Source: CAD feature listing. Evaluate the final solid. Frame: model axes, mm. Round coordinates to 2 decimals unless told otherwise and drop trailing zeros. Order: outer loops, then holes, each group sorted by start corner. A loop starts at its lowest first (then second) coordinate and runs counter-clockwise, first axis right, second up. Notation, with made-up numbers: (-28.75, -31.75) - (22.25, -31.75) arc R14 ccw to (22.25, -10.75) - close; hole circle Ø3 at (-38.75, 68.5). An arc over 180 degrees is marked (long way). Use one line per item in the form item = value. Start each with the question number.
Q1. Cut plane A-A, the plane y = 4.25. Return the cut outline in (x, z).
Q2. Ray query, line 1 (X direction, y = 16, z = -608); line 2 (Z direction, x = 79.5, y = 10.5); line 3 (X direction, y = 16.75, z = -755). Return the intervals inside material, ascending. Write a range as [from, to].
Q3. Pin query (flat end, axial travel): pin 1 Ø8 at (y, z) = (16, -914.5) entering from -X; pin 2 Ø4 at (x, z) = (-200.03, -287.05) entering from -Y; pin 3 Ø2 at (y, z) = (5.5, -580) entering from -X; pin 4 Ø8 at (x, y) = (-276.5, 5.5) entering from +Z. Return the tip coordinate at first contact, or that it passes through.
Q4. Cut plane B-B, the plane x = -234.5. Return the cut outline in (y, z).
from build123d import *

# Parameters (mm, degrees)
BOSS_EXTRUDE3_DEPTH = 19.05
SKETCH6_R           = 3.175
CUT_EXTRUDE3_DEPTH  = 9.525
CUT_EXTRUDE4_DEPTH  = 9.525


with BuildPart() as part:
    # Sketch2 → Boss-Extrude3 (new body)
    with BuildSketch(Plane(origin=(0, 0, 0), x_dir=(1, 0, 0), z_dir=(0, 1, 0))):
        Polygon((-336.69350738, 0), (-316.143895572, 0), (-209.015455166, 264.828592555), (-221.216787177, 285.466092555), align=None)
        Polygon((-316.143895572, 0), (-295.594283764, 0), (-196.814123155, 244.191092555), (-209.015455166, 264.828592555), align=None)
        with BuildLine():
            Line((-322.659375, -16.106696225), (-316.143895572, 0))
            Line((-316.143895572, 0), (-336.69350738, 0))
            Line((-336.69350738, 0), (-341.509822647, -11.90625))
            Line((-341.509822647, -11.90625), (-326.793303775, -17.859375))
            ThreePointArc((-326.793303775, -17.859375), (-325.089331047, -16.126870931), (-322.659375, -16.106696225))
        make_face()
        with BuildLine():
            Line((-303.300388192, -19.05), (-295.594283764, 0))
            Line((-295.594283764, 0), (-316.143895572, 0))
            Line((-316.143895572, 0), (-322.659375, -16.106696225))
            ThreePointArc((-322.659375, -16.106696225), (-321.217429073, -17.275121043), (-320.675, -19.05))
            Line((-320.675, -19.05), (-303.300388192, -19.05))
        make_face()
        with BuildLine():
            Line((-327.557139607, -38.1), (-311.00649262, -38.1))
            Line((-311.00649262, -38.1), (-306.190177353, -26.19375))
            Line((-306.190177353, -26.19375), (-320.906696225, -20.240625))
            ThreePointArc((-320.906696225, -20.240625), (-325.040625, -21.993303775), (-326.793303775, -17.859375))
            Line((-326.793303775, -17.859375), (-341.509822647, -11.90625))
            Line((-341.509822647, -11.90625), (-348.653572647, -29.566072647))
            Line((-348.653572647, -29.566072647), (-327.557139607, -38.1))
        make_face()
        with BuildLine():
            Line((-320.906696225, -20.240625), (-306.190177353, -26.19375))
            Line((-306.190177353, -26.19375), (-303.300388192, -19.05))
            Line((-303.300388192, -19.05), (-320.675, -19.05))
            ThreePointArc((-320.675, -19.05), (-320.733462299, -19.656479808), (-320.906696225, -20.240625))
        make_face()
        Polygon((-313.333927353, -43.853572647), (-311.00649262, -38.1), (-327.557139607, -38.1), align=None)
        Polygon((-183.626593256, 296.748681841), (-178.833212823, 288.641092555), (143.866072647, 1086.375076786), (108.546427353, 1100.662576786), (-215.267964049, 300.171976915), (-193.321682542, 313.147088585), align=None)
        with BuildLine():
            Line((-196.814123155, 244.191092555), (-187.823667989, 266.416092555))
            Line((-187.823667989, 266.416092555), (-198.409151786, 284.320524764))
            ThreePointArc((-198.409151786, 284.320524764), (-199.787821823, 283.887463765), (-201.215625, 284.11028878))
            Line((-201.215625, 284.11028878), (-209.015455166, 264.828592555))
            Line((-209.015455166, 264.828592555), (-196.814123155, 244.191092555))
        make_face()
        with BuildLine():
            Line((-197.291932209, 288.669440769), (-183.626593256, 296.748681841))
            Line((-183.626593256, 296.748681841), (-193.321682542, 313.147088585))
            Line((-193.321682542, 313.147088585), (-215.267964049, 300.171976915))
            Line((-215.267964049, 300.171976915), (-221.216787177, 285.466092555))
            Line((-221.216787177, 285.466092555), (-209.015455166, 264.828592555))
            Line((-209.015455166, 264.828592555), (-201.215625, 284.11028878))
            ThreePointArc((-201.215625, 284.11028878), (-202.431501435, 289.124673395), (-197.291932209, 288.669440769))
        make_face()
        with BuildLine():
            Line((-187.823667989, 266.416092555), (-178.833212823, 288.641092555))
            Line((-178.833212823, 288.641092555), (-183.626593256, 296.748681841))
            Line((-183.626593256, 296.748681841), (-197.291932209, 288.669440769))
            ThreePointArc((-197.291932209, 288.669440769), (-196.962475287, 287.891188748), (-196.85, 287.053592555))
            ThreePointArc((-196.85, 287.053592555), (-197.26719806, 285.480330511), (-198.409151786, 284.320524764))
            Line((-198.409151786, 284.320524764), (-187.823667989, 266.416092555))
        make_face()
    extrude(amount=BOSS_EXTRUDE3_DEPTH)

    # Sketch6 → Cut-Extrude3 (cut)
    with BuildSketch(Plane.XZ):
        Polygon((-327.557139607, 38.1), (-348.653572647, 29.566072647), (-336.69350738, 0), (-295.594283764, 0), (-311.00649262, 38.1), align=None)
        with Locations(Location((-323.85, 19.05, 0), (0, 0, 270))):
            Circle(SKETCH6_R, mode=Mode.SUBTRACT)
    extrude(amount=-CUT_EXTRUDE3_DEPTH, mode=Mode.SUBTRACT)

    # Sketch7 → Cut-Extrude4 (cut)
    with BuildSketch(Plane.XZ):
        Polygon((-196.814123155, -244.191092555), (-221.216787177, -285.466092555), (-215.267964049, -300.171976915), (-193.321682542, -313.147088585), (-178.833212823, -288.641092555), align=None)
    extrude(amount=-CUT_EXTRUDE4_DEPTH, mode=Mode.SUBTRACT)


solid = part.part
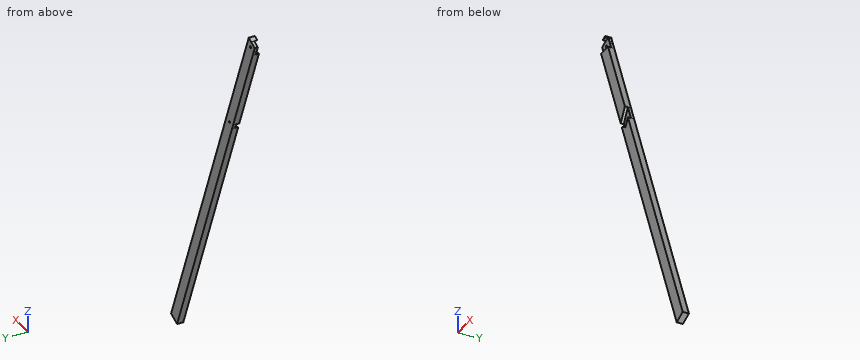
Completed:
q1.outline = (-336.69, 0) - (-221.22, -285.47) - (-196.81, -244.19) - (-295.59, 0) - close; (-327.56, 38.1) - (-311.01, 38.1) - (-313.33, 43.85) - close; (-215.27, -300.17) - (108.55, -1100.66) - (143.87, -1086.38) - (-178.83, -288.64) - (-193.32, -313.15) - close
q2.line_1 = [-90.75, -49.65]
q2.line_2 = [-1028.86, -927.26]
q2.line_3 = [-31.28, 9.82]
q3.pin_1 = 31.62
q3.pin_2 = through
q3.pin_3 = -102.48
q3.pin_4 = -37.31
q4.outline = (0, -252.63) - (19.05, -252.63) - (19.05, -151.03) - (0, -151.03) - close
